from build123d import *

# Parameters (mm, degrees)
CROQUIS1_R              = 1.25
SALIENTE_EXTRUIR1_DEPTH = 1.75


with BuildPart() as part:
    # Croquis1 → Saliente-Extruir1 (new body)
    with BuildSketch(Plane.XY.offset(1.75)):
        with BuildLine():
            Line((5.249381166, 19.859670123), (4.53882245, 18.144188898))
            ThreePointArc((4.53882245, 18.144188898), (5.400610321, 14.913797401), (8.743959767, 14.902750233))
            ThreePointArc((8.743959767, 14.902750233), (10.704311129, 15.511176573), (12.596981786, 14.716848016))
            ThreePointArc((12.596981786, 14.716848016), (0, -17.45), (-12.596981786, 14.716848016))
            ThreePointArc((-12.596981786, 14.716848016), (-10.704311129, 15.511176573), (-8.743959767, 14.902750233))
            ThreePointArc((-8.743959767, 14.902750233), (-5.400610321, 14.913797401), (-4.53882245, 18.144188898))
            Line((-4.53882245, 18.144188898), (-5.249381166, 19.859670123))
            ThreePointArc((-5.249381166, 19.859670123), (-5.64740484, 20.277175016), (-6.222755816, 20.318459835))
            ThreePointArc((-6.222755816, 20.318459835), (0, -21.25), (6.222755816, 20.318459835))
            ThreePointArc((6.222755816, 20.318459835), (5.64740484, 20.277175016), (5.249381166, 19.859670123))
        make_face()
        with Locations(Location((-7.0795, 17.09183079, 0), (0, 0, 180))):
            Circle(CROQUIS1_R, mode=Mode.SUBTRACT)
        with Locations(Location((7.0795, 17.09183079, 0), (0, 0, 180))):
            Circle(CROQUIS1_R, mode=Mode.SUBTRACT)
    extrude(amount=-SALIENTE_EXTRUIR1_DEPTH)


solid = part.part
Work out the finished part from the listing and answer in its coordinate system (mm). A direction names the side the tool comes from. Round coordinates to 2 decimals unless told otherwise and drop trailing zeros. Order: outer loops, then holes, each group sorted by start corner. A loop starts at its lowest first (then second) coordinate and runs counter-clockwise, first axis right, second up. Notation, with made-up numbers: M 38.25,43.5 L 73.25,43.5 A31 cw 73.25,81.5 Z; hole C 67,87.25 d6. An arc over 180 degrees is marked long. Put each result on its own line as item: value. Start each with the question number.
Q1. Section D-D, the plane x = 0 is taken. Write down the section's boundary in (y, z).
Q2. Section C-C, the plane z = 0.9 is taken. Write down the section's boundary in (x, y), and give its area (3 significant figures).
Q3. A tool of negligible diameter and unlimited length cuts with its end or side. For faces 1 (the cylindrical face through (-10.73, 15.51, 0.89)), 2 (the flat face through (4.899, 19.014, 0.887)), 3 (the flat face through (-5, -17, 1.75)), from which of +Z, -Z, +X, -X, +Y, -Y can it reach the whole face along a straight path? Write none if from no direction.
Q4. For a pull along Y with two mould halves and no side action, classify faces 4 (the cylindrical face through (5.7, 20.3, 0.9)), 5 (the flat face through (-5, -17, 0)), 6 (the cylindrical face through (-0.846, -21.233, 0.887)), 7 (the cylindrical face through (-5.441, 14.883, 0.887)) as pulls with the +Y half, pulls with the -Y half, needs draft (parallel to the pull), parting line crosses it, or undercut.
Q5. Section B-B, the plane y = 1.1 is taken. Write down the section's boundary in (x, z).
Q6. Straight lines are drawn through the part: L1, parallel to Y at x = -7.5, z = 1.15; L2, parallel to X at y = 18, z = 0.8; L3, parallel to Y at x = 6, z = 1.55. For each, find the intervals that lie inside material, in ascending order. Write a range as [from, to].
Q7. Section A-A, the plane x = 12 is taken. Write down the section's boundary in (y, z), and give its area (3 significant figures).
Findings below:
1. outline: M -21.25,0 L -17.45,0 L -17.45,1.75 L -21.25,1.75 Z
2. outline: M -12.6,14.72 A3 cw -8.74,14.9 A2.75 ccw -4.54,18.14 L -5.25,19.86 A0.8 ccw -6.22,20.32 A21.25 ccw long 6.22,20.32 A0.8 ccw 5.25,19.86 L 4.54,18.14 A2.75 ccw 8.74,14.9 A3 cw 12.6,14.72 A18.55 cw long Z; hole C -7.08,17.09 d2.5; hole C 7.08,17.09 d2.5
2. area: 349 mm^2
3. face 1: +Z, -Z
3. face 2: +Z, -Z, +Y
3. face 3: +Z, +X, -X, +Y, -Y
4. face 4: pulls with the +Y half
4. face 5: needs draft
4. face 6: parting line crosses it
4. face 7: undercut
5. outline: M -21.22,0 L -18.55,0 L -18.55,1.75 L -21.22,1.75 Z; M 18.55,0 L 21.22,0 L 21.22,1.75 L 18.55,1.75 Z
6. L1: y = [-19.88, -15.87], [14.37, 15.91], [18.27, 19.88]
6. L2: x = [-11.29, -7.94], [-6.22, -4.48], [4.48, 6.22], [7.94, 11.29]
6. L3: y = [-20.39, -16.45], [14.56, 16.46], [17.72, 20.35]
7. outline: M -17.54,0 L -13.05,0 L -13.05,1.75 L -17.54,1.75 Z; M 15.15,0 L 17.54,0 L 17.54,1.75 L 15.15,1.75 Z
7. area: 12.0 mm^2
